Can you work these out from the drawing? Everything is in mm from the part's minimum corner. A direction names the side the tool comes from. Round coordinates to 2 decimals unless told otherwise and drop trailing zeros. Loops run counter-clockwise (first coordinate to the right, second up) from the corner with the lowest first, then second, coordinate; pieces in that order, holes last. Notation, with made-up numbers: M -34.5,21 L 14.5,21 A20 cw 14.5,33 Z; hole C 63,52 d4. An arc over 180 degrees is marked long. Answer in a Markdown table with one row per item.
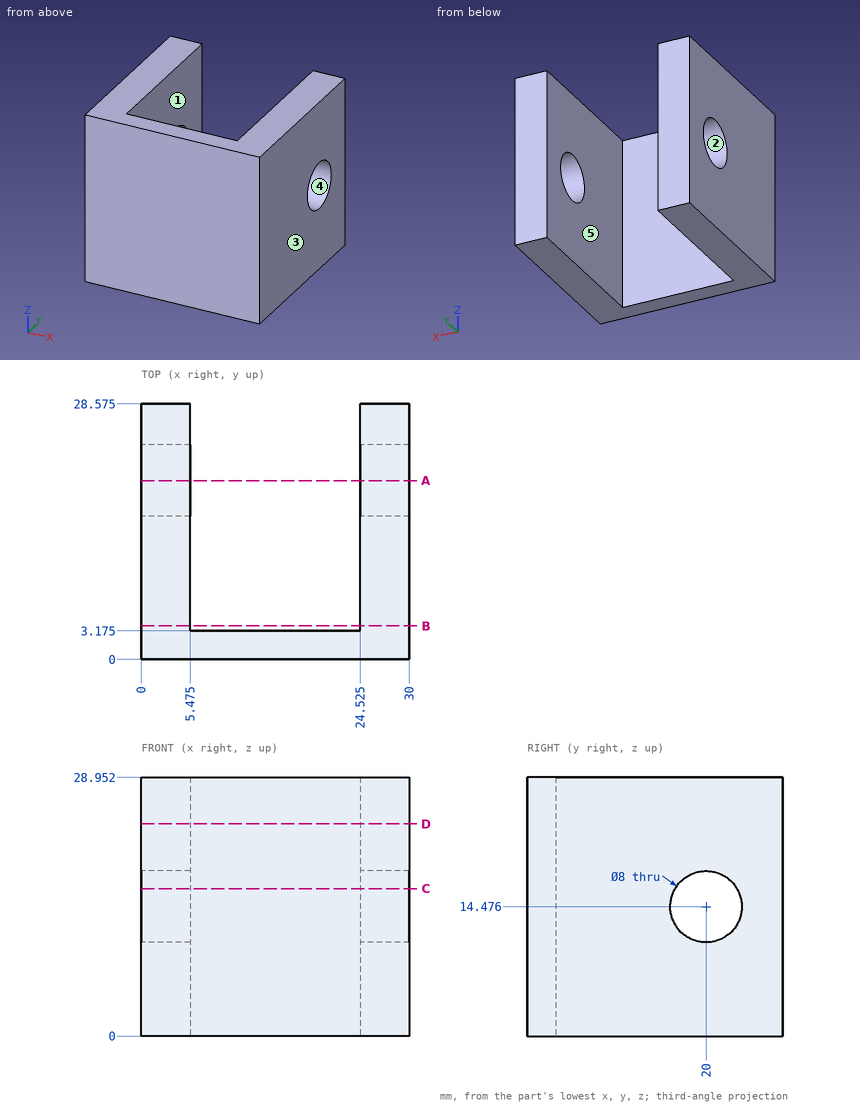
1) I want a section at A-A, the plane y = 20. Please give me the cut outline in (x, z) (1 decimal).
Computed:
| item | result |
|---|---|
| outline | M 0,0 L 5.5,0 L 5.5,10.5 L 0,10.5 Z; M 0,18.5 L 5.5,18.5 L 5.5,29 L 0,29 Z; M 24.5,0 L 30,0 L 30,10.5 L 24.5,10.5 Z; M 24.5,18.5 L 30,18.5 L 30,29 L 24.5,29 Z |
2) I want a section at B-B, the plane y = 3.75. Please give me the cut outline in (x, z) (1 decimal).
Computed:
| item | result |
|---|---|
| outline | M 0,0 L 5.5,0 L 5.5,29 L 0,29 Z; M 24.5,0 L 30,0 L 30,29 L 24.5,29 Z |
3) If we mould it in two halves opening along X, with no side actions, what happens to the marked faces 1, 2 and 3? For each: released by +X, released by -X, zero draft, split by the parting line, or undercut.
Computed:
| item | result |
|---|---|
| face 1 | undercut |
| face 2 | zero draft |
| face 3 | released by +X |
4) I want a section at D-D, the plane z = 23.75. Please give me the cut outline in (x, y) (1 decimal).
Computed:
| item | result |
|---|---|
| outline | M 0,0 L 30,0 L 30,28.6 L 24.5,28.6 L 24.5,3.2 L 5.5,3.2 L 5.5,28.6 L 0,28.6 Z |
5) Which directions (+Z, -Z, +X, -X, +Y, -Y) give clear straight access to the entire face, cutting with the end or side of a thin tool? Please do the marked faces 4 and 5.
Computed:
| item | result |
|---|---|
| face 4 | +X, -X |
| face 5 | +Z, -Z, +Y |
6) I want a section at C-C, the plane z = 16.5. State how many separate pieces and enclosed holes the cut face has, plus the area to 3 significant figures.
Computed:
| item | result |
|---|---|
| separate pieces | 3 |
| enclosed holes | 0 |
| area | 298 mm² |
7) I need wall thicknesses on line 1 (X direction, y = 19.75, z = 26.5) (1 decimal); line 2 (Z direction, x = 1.45, y = 20); line 3 (Y direction, x = 16.5, z = 27.75) (1 decimal). Which ranges of each line are inside material? Lowest first, please.
Computed:
| item | result |
|---|---|
| line 1 | x = 0 to 5.5, 24.5 to 30 |
| line 2 | z = 0 to 10.48, 18.48 to 28.95 |
| line 3 | y = 0 to 3.2 |
8) Will this pin go through, and if not, where does the flat tip stop? P1, Ø3, axis at y = 18, z = 15.5, coming from the -X side.
Computed:
| item | result |
|---|---|
| P1 | passes through |
